Autodesk Inventor part; units mm, degrees
ref_plane "YZ Plane" through (0, 0, 0) normal (1, 0, 0) x (0, 1, 0)
ref_plane "XZ Plane" through (0, 0, 0) normal (0, 1, 0) x (-1, 0, 0)
ref_plane "XY Plane" through (0, 0, 0) normal (0, 0, 1) x (1, 0, 0)
sketch "Sketch1" plane through (0, 0, 0) normal (0, 0, 1) x (1, 0, 0)
  line L0 (-43.5443, 19.427) -> (49.4557, 19.427)
  line L1 (52.4557, 16.427) -> (52.4557, -43.573)
  line L2 (49.4557, -46.573) -> (-43.5443, -46.573)
  line L3 (-46.5443, -43.573) -> (-46.5443, 16.427)
  arc A0 (-43.5443, 19.427) -> (-46.5443, 16.427) centre (-43.5443, 16.427) ccw
  arc A1 (-46.5443, -43.573) -> (-43.5443, -46.573) centre (-43.5443, -43.573) ccw
  arc A2 (49.4557, -46.573) -> (52.4557, -43.573) centre (49.4557, -43.573) ccw
  arc A3 (52.4557, 16.427) -> (49.4557, 19.427) centre (49.4557, 16.427) ccw
  point P0 (0, 0)
  point P1 (0, 0)
  point P2 (-46.5443, 19.427)
  point P3 (52.4557, -46.573)
  point P4 (52.4557, 19.427)
  dimension "d0" = 99
  dimension "d1" = 66
  dimension "d2" = 3
extrude "Extrusion1" add sketch "Sketch1" along normal blind 12.7
sketch "Sketch2" plane through (0, 0, 12.7) normal (0, 0, 1) x (1, 0, 0)
  line L0 (-46.5443, 16.427) -> (-46.5443, -43.573)
  line L1 (49.4557, 19.427) -> (-43.5443, 19.427)
  circle A0 centre (-42.7343, 15.617) radius 1.905
  line L2 (-50.0562, -13.573) -> (79.0191, -13.573) construction
  line L3 (2.9557, 30.2203) -> (2.9557, -48.7988) construction
  circle A1 centre (-42.7343, -42.763) radius 1.905
  circle A2 centre (48.6457, 15.617) radius 1.905
  circle A3 centre (48.6457, -42.763) radius 1.905
  point P0 (0, 0)
  dimension "d8" = 3.81
  dimension "d9" = 3.81
  dimension "d10" = 3.81
  dimension "d50" = 3.81
  dimension "d51" = 3.81
  dimension "d52" = 3.81
extrude "Extrusion2" cut sketch "Sketch2" against normal blind 25.4
sketch "Sketch3" plane through (0, 0, 12.7) normal (0, 0, 1) x (1, 0, 0)
  circle A0 centre (48.6457, 15.617) radius 1.905
  circle A1 centre (-42.7343, 15.617) radius 1.905
  circle A2 centre (-42.7343, -42.763) radius 1.905
  circle A3 centre (48.6457, -42.763) radius 1.905
  line L0 (49.4557, 19.427) -> (-43.5443, 19.427)
  arc A4 (-43.5443, 19.427) -> (-46.5443, 16.427) centre (-43.5443, 16.427) ccw
  line L1 (-46.5443, 16.427) -> (-46.5443, -43.573) construction
  arc A5 (-46.5443, -43.573) -> (-43.5443, -46.573) centre (-43.5443, -43.573) ccw
  line L2 (-43.5443, -46.573) -> (49.4557, -46.573)
  arc A6 (49.4557, -46.573) -> (52.4557, -43.573) centre (49.4557, -43.573) ccw
  line L3 (52.4557, -43.573) -> (52.4557, 16.427)
  arc A7 (52.4557, 16.427) -> (49.4557, 19.427) centre (49.4557, 16.427) ccw
  arc A8 (-43.5443, 19.427) -> (-46.5443, 16.427) centre (-43.5443, 16.427) ccw
  line L4 (49.4557, 19.427) -> (-43.5443, 19.427)
  circle A9 centre (48.6457, 15.617) radius 1.905
  circle A10 centre (-42.7343, 15.617) radius 1.905
  circle A11 centre (-42.7343, -42.763) radius 1.905
  circle A12 centre (48.6457, -42.763) radius 1.905
  arc A13 (52.4557, 16.427) -> (49.4557, 19.427) centre (49.4557, 16.427) ccw
  line L5 (52.4557, 16.427) -> (52.4557, -43.573)
  arc A14 (49.4557, -46.573) -> (52.4557, -43.573) centre (49.4557, -43.573) ccw
  line L6 (49.4557, -46.573) -> (-43.5443, -46.573)
  arc A15 (-46.5443, -43.573) -> (-43.5443, -46.573) centre (-43.5443, -43.573) ccw
  line L7 (-46.5443, -43.573) -> (-46.5443, 16.427)
  arc A16 (-43.5443, 19.427) -> (-46.5443, 16.427) centre (-43.5443, 16.427) ccw
  line L8 (-43.5443, 19.427) -> (49.4557, 19.427)
  line L9 (-43.5443, 19.427) -> (49.4557, 19.427)
  line L10 (-40.8039, 19.427) -> (-40.8039, -46.573) construction
  line L11 (49.4557, -46.573) -> (-43.5443, -46.573)
  line L12 (-40.8039, 19.427) -> (-51.3078, 19.427) construction
  line L13 (-40.8039, -46.573) -> (-51.3078, -46.573) construction
  line L14 (-40.8039, -21.173) -> (-51.3078, -21.173) construction
  line L15 (-40.8039, -5.973) -> (-51.3078, -5.973) construction
  line L16 (-46.5443, -43.573) -> (-46.5443, 16.427)
  line L17 (-46.5443, -5.973) -> (-40.8039, -5.973)
  line L18 (-40.8039, -5.973) -> (-40.8039, -21.173)
  line L19 (-40.8039, -21.173) -> (-46.5443, -21.173)
  line L20 (-46.5443, -21.173) -> (-46.5443, -5.973)
  point P0 (0, 0)
  dimension "d13" = 25.4
  dimension "d14" = 25.4
  dimension "d15" = 5.7404
extrude "Extrusion3" cut sketch "Sketch3" against normal blind 25.4 contours L17 L18 L19 L7
fillet "Fillet1" radius 3.175 2 edges at (-46.5443, -21.173, 6.35) (-46.5443, -5.973, 6.35)
sketch "Sketch9" plane through (0, 0, 12.7) normal (0, 0, 1) x (1, 0, 0)
  arc A0 (-43.5443, 19.427) -> (-46.5443, 16.427) centre (-43.5443, 16.427) ccw
  line L0 (-46.5443, -2.798) -> (-46.5443, 16.427) construction
  line L1 (-46.5443, 16.427) -> (-46.5443, -2.798)
  line L2 (-43.5443, 19.427) -> (-26.5771, 19.427) construction
  line L3 (49.4557, 19.427) -> (-43.5443, 19.427)
  line L4 (-45.6657, 18.5483) -> (-26.5771, -0.5403) construction
  line L5 (-45.6657, 18.5483) -> (-18.6704, 18.5483) construction
  circle A1 centre (-45.6657, 18.5483) radius 7.1603
  arc A2 (-46.5443, -2.798) -> (-43.3693, -5.973) centre (-43.3693, -2.798) ccw
  line L6 (-43.3693, -5.973) -> (-40.8039, -5.973)
  line L7 (-40.8039, -5.973) -> (-40.8039, -21.173)
  line L8 (-40.8039, -21.173) -> (-43.3693, -21.173)
  arc A3 (-43.3693, -21.173) -> (-46.5443, -24.348) centre (-43.3693, -24.348) ccw
  line L9 (-46.5443, -24.348) -> (-46.5443, -43.573)
  arc A4 (-46.5443, -43.573) -> (-43.5443, -46.573) centre (-43.5443, -43.573) ccw
  line L10 (-43.5443, -46.573) -> (49.4557, -46.573)
  arc A5 (49.4557, -46.573) -> (52.4557, -43.573) centre (49.4557, -43.573) ccw
  line L11 (52.4557, -43.573) -> (52.4557, 16.427)
  arc A6 (52.4557, 16.427) -> (49.4557, 19.427) centre (49.4557, 16.427) ccw
  line L12 (49.4557, 19.427) -> (-43.5443, 19.427)
  arc A7 (-43.5443, 19.427) -> (-46.5443, 16.427) centre (-43.5443, 16.427) ccw
  line L13 (-46.5443, 16.427) -> (-46.5443, -2.798)
  circle A8 centre (48.6457, 15.617) radius 1.905
  circle A9 centre (-42.7343, 15.617) radius 1.905
  circle A10 centre (-42.7343, -42.763) radius 1.905
  circle A11 centre (48.6457, -42.763) radius 1.905
  line L14 (-75.7777, -13.573) -> (114.1059, -13.573) construction
  line L15 (2.9557, 31.1348) -> (2.9557, -53.319) construction
  circle A12 centre (-45.6657, -45.6944) radius 7.1603
  line L16 (2.9557, -58.2809) -> (2.9557, 26.1729) construction
  circle A13 centre (51.577, 18.5483) radius 7.1603
  circle A14 centre (51.577, -45.6944) radius 7.1603
  point P0 (0, 0)
  dimension "d28" = 45
extrude "Extrusion5" cut sketch "Sketch9" against normal blind 11.43 contours L3 A1 L1 A0 | A0 L1 A1 L3 | A13 L11 A6 L3 | L3 A6 L11 A13 | A14 L10 A5 L11 | L11 A5 L10 A14 | A12 L9 A4 L10 | L10 A4 L9 A12
sketch "Sketch10" plane through (0, 0, 12.7) normal (0, 0, 1) x (1, 0, 0)
  arc A0 (52.4557, -38.5882) -> (44.4708, -46.573) centre (51.577, -45.6944) ccw
  line L0 (52.4557, -38.5882) -> (52.4557, 11.4421)
  arc A1 (44.4708, 19.427) -> (52.4557, 11.4421) centre (51.577, 18.5483) ccw
  line L1 (44.4708, 19.427) -> (-38.5595, 19.427)
  arc A2 (-46.5443, 11.4421) -> (-38.5595, 19.427) centre (-45.6657, 18.5483) ccw
  line L2 (-46.5443, 11.4421) -> (-46.5443, -2.798)
  arc A3 (-46.5443, -2.798) -> (-43.3693, -5.973) centre (-43.3693, -2.798) ccw
  line L3 (-43.3693, -5.973) -> (-40.8039, -5.973)
  line L4 (-40.8039, -5.973) -> (-40.8039, -21.173)
  line L5 (-40.8039, -21.173) -> (-43.3693, -21.173)
  arc A4 (-43.3693, -21.173) -> (-46.5443, -24.348) centre (-43.3693, -24.348) ccw
  line L6 (-46.5443, -24.348) -> (-46.5443, -38.5882)
  arc A5 (-38.5595, -46.573) -> (-46.5443, -38.5882) centre (-45.6657, -45.6944) ccw
  line L7 (-38.5595, -46.573) -> (44.4708, -46.573)
  line L8 (-36.7645, -45.303) -> (43.1467, -45.303)
  line L9 (-36.7645, 18.157) -> (43.1467, 18.157)
  line L10 (44.4708, 19.427) -> (-38.5595, 19.427)
  line L11 (-36.7645, -45.303) -> (-37.2353, -45.303)
  arc A6 (-38.5595, -46.573) -> (-46.5443, -38.5882) centre (-45.6657, -45.6944) ccw
  line L12 (-36.7645, 18.157) -> (-37.2353, 18.157)
  line L13 (51.1857, 10.118) -> (51.1857, -37.264)
  arc A7 (44.4708, 19.427) -> (52.4557, 11.4421) centre (51.577, 18.5483) ccw
  line L14 (-39.5339, -5.973) -> (-39.5339, -21.173)
  line L15 (-45.2743, -2.798) -> (-39.5339, -5.973)
  line L16 (-39.5339, -21.173) -> (-45.2743, -24.348)
  line L17 (51.1857, 10.118) -> (52.4557, 10.118) construction
  line L18 (52.4557, -38.5882) -> (52.4557, 11.4421)
  line L19 (43.1467, 18.157) -> (43.1467, 19.427) construction
  arc A8 (43.1467, 18.157) -> (51.1857, 10.118) centre (51.577, 18.5483) ccw
  line L20 (-56.5649, -13.573) -> (80.9191, -13.573) construction
  line L21 (2.9557, 34.2968) -> (2.9557, -68.6615) construction
  arc A9 (51.1857, -37.264) -> (43.1467, -45.303) centre (51.577, -45.6944) ccw
  arc A10 (-45.2743, 10.118) -> (-37.2353, 18.157) centre (-45.6657, 18.5483) ccw
  arc A11 (-37.2353, -45.303) -> (-45.2743, -37.264) centre (-45.6657, -45.6944) ccw
  line L22 (-45.2743, 10.118) -> (-45.2743, -2.798)
  line L23 (-45.2743, -37.264) -> (-45.2743, -24.348)
  line L24 (-46.5443, -43.573) -> (-46.5443, -24.348)
  point P0 (0, 0)
  dimension "d31" = 1.27
  dimension "d32" = 1.27
  dimension "d35" = 1.27
  dimension "d36" = 1.27
  dimension "d39" = 3.175
  dimension "d40" = 3.175
  dimension "d42" = 1.27
  dimension "d43" = 1.27
  dimension "d44" = 1.2791
extrude "Extrusion6" cut sketch "Sketch10" against normal blind 11.43 contours L11 A11 L23 L16 L14 L15 L22 A10 L12 L9 A8 L13 A9 L8
sketch "Sketch11" plane through (-40.8039, -21.173, 12.7) normal (-1, 0, 0) x (0, 0, 1)
  line L0 (-12.7, 0) -> (-12.7, 15.2)
  line L1 (0, 0) -> (-12.7, 0)
  line L2 (0, 15.2) -> (0, 0)
  line L3 (0, 15.2) -> (-12.7, 15.2)
  line L4 (-11.43, 0) -> (-11.43, 15.2)
  line L5 (0, 15.2) -> (-11.43, 15.2)
  line L6 (0, 0) -> (-11.43, 0)
  line L7 (0, 15.2) -> (-11.43, 15.2)
  line L8 (-11.43, 15.2) -> (-11.43, 0)
  line L9 (-11.43, 0) -> (0, 0)
  line L10 (0, 0) -> (0, 15.2)
  point P0 (-12.7, 21.173)
extrude "Extrusion7" cut sketch "Sketch11" against normal blind 7.62 contours L4 L3 L2 L1
fillet "Fillet2" radius 3.175 2 edges at (-39.5339, -21.173, 6.985) (-39.5339, -5.973, 6.985)
properties part number "battbase_final"
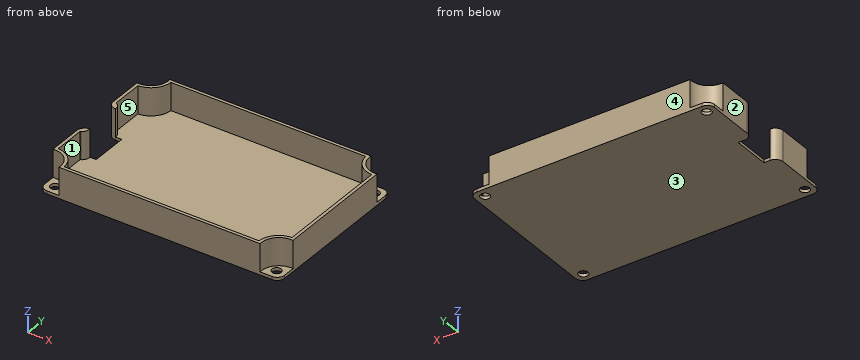
Part model, mm, in its own coordinate system. Face numbers are marked on the shaded views. A direction names the side the tool comes from. Round coordinates to 2 decimals unless told otherwise and drop trailing zeros. Write each loop counter-clockwise with the first axis right and the second up, starting at its lowest first coordinate (ties: lowest second). Pieces come first, ordered by that corner, then holes. Notation, with made-up numbers: M 37.5,-2 L 46.5,-2 A24 cw 46.5,8 Z; hole C 36,33 d1. An arc over 180 degrees is marked long. One line per question, with ' | ' between items.
(1) Saw through at D-D on y = -18. Write the cut outline in (x, z), then the cut area to 3 significant figures.
Answer key:
outline: M -40.8,0 L 52.46,0 L 52.46,12.7 L 51.19,12.7 L 51.19,1.27 L -40.8,1.27 Z | area: 133 mm^2
(2) Probe line 1 along X through (y, z) = (-35, 7.5); line 2 along Y through (x, z) = (-19, 9.25); line 3 along Z through (x, y) = (-13.5, 4). List the from-to ranges inside material, lowest first.
Answer key:
line 1: x = -46.54 to -45.27, 51.19 to 52.46 | line 2: y = -46.57 to -45.3, 18.16 to 19.43 | line 3: z = 0 to 1.27
(3) Two-plate mould, pull along X, no slides. Class the marked faces 1, 2 and 3: released by +X, released by -X, zero draft, split by the parting line, or undercut.
Answer key:
face 1: undercut | face 2: released by -X | face 3: zero draft
(4) Saw through at A-A on y = -36. Write the cut outline in (x, z).
Answer key:
outline: M -46.54,0 L 52.46,0 L 52.46,12.7 L 51.19,12.7 L 51.19,1.27 L -45.27,1.27 L -45.27,12.7 L -46.54,12.7 Z
(5) 3-axis set-ups, long thin cutter, end or side, ignore diameter. For the marked faces 4 and 5: which of +Z, -Z, +X, -X, +Y, -Y reach the whole face in a straight line?
Answer key:
face 4: +Z, -Z, +X, -X, +Y | face 5: +Z
(6) Pin check, flat tip, straight feed: pin 1 (4 mm diameter, centred on x = -43, y = 15, fed in from +Z). Stop position of the tip, or through.
Answer key:
pin 1: stops at z = 1.27
(7) Saw through at B-B on x = 14.5. Write the cut outline in (y, z).
Answer key:
outline: M -46.57,0 L 19.43,0 L 19.43,12.7 L 18.16,12.7 L 18.16,1.27 L -45.3,1.27 L -45.3,12.7 L -46.57,12.7 Z
